```python
from build123d import *

# Parameters (mm, degrees)
BOSS_EXTRUDE1_DEPTH = 25
SKETCH2_OUTSIDE_W   = 63.85
SKETCH2_OUTSIDE_H   = 61.22
SKETCH2_OUTSIDE_R   = 8.5
CUT_EXTRUDE1_DEPTH  = 25
CUT_EXTRUDE1_DRAFT  = -35
SKETCH3_R           = 6
BOSS_EXTRUDE2_DEPTH = 110
SKETCH4_R           = 4
BOSS_EXTRUDE3_DEPTH = 6


with BuildPart() as part:
    # Sketch1 → Boss-Extrude1 (new body)
    with BuildSketch(Plane(origin=(0, 0, 0), x_dir=(1, 0, 0), z_dir=(0, 1, 0))):
        Polygon((9.814954576, 0), (4.907477288, 8.5), (-4.907477288, 8.5), (-9.814954576, 0), (-4.907477288, -8.5), (4.907477288, -8.5), align=None)
    extrude(amount=-BOSS_EXTRUDE1_DEPTH)


with BuildPart() as cut_extrude1_tool:
    # Sketch2 outside → Cut-Extrude1 (with draft: the straight prism first)
    with BuildSketch(Plane(origin=(0, 0, 0), x_dir=(1, 0, 0), z_dir=(0, 1, 0))):
        Rectangle(SKETCH2_OUTSIDE_W, SKETCH2_OUTSIDE_H)
        Circle(SKETCH2_OUTSIDE_R, mode=Mode.SUBTRACT)
    extrude(amount=-CUT_EXTRUDE1_DEPTH)
    # Cut-Extrude1: the draft: its side faces are tilted about the plane it starts from
    cut_extrude1_sides = [cut_extrude1_tool.faces().sort_by_distance(p)[0] for p in [
        (0, -12.5, 30.61),
        (31.925, -12.5, 0),
        (0, -12.5, -30.61),
        (-31.925, -12.5, 0),
        (-8.5, -12.5, 0),
    ]]
    draft(cut_extrude1_sides, Plane(origin=(0, 0, 0), x_dir=(1, 0, 0), z_dir=(0, 1, 0)), CUT_EXTRUDE1_DRAFT)


with BuildPart() as part_1:
    add(part.part)

    # Cut-Extrude1: cut by cut_extrude1_tool
    add(cut_extrude1_tool.part, mode=Mode.SUBTRACT)

    # Sketch3 → Boss-Extrude2 (add)
    with BuildSketch(Plane.XZ.offset(25)):
        with Locations(Location((0, 0, 0), (0, 0, 90))):
            Circle(SKETCH3_R)
    extrude(amount=BOSS_EXTRUDE2_DEPTH)

    # Sketch4 → Boss-Extrude3 (add)
    with BuildSketch(Plane.XZ.offset(135)):
        with Locations(Location((0, 0, 0), (0, 0, 270))):
            Circle(SKETCH4_R)
    extrude(amount=BOSS_EXTRUDE3_DEPTH)

    # Boss-Extrude4 cone 1 section (through the dimple's axis) → Boss-Extrude4 (revolve)
    with BuildSketch(Plane(origin=(0, -141, 0), x_dir=(0, 0, 1), z_dir=(1, 0, 0))):
        Polygon((0, 0), (4, 0), (0, 4), align=None)
    revolve(axis=Axis((0, -141, 0), (0, -1, 0)))


solid = part_1.part
```
Read the model definition and answer for the solid it produces. Units are mm, in the model's axes. A direction names the side the tool comes from. Give positions to 0.01 mm unless a question says otherwise; leave off trailing zeros. Write each loop counter-clockwise with the first axis right and the second up, starting at its lowest first coordinate (ties: lowest second). Pieces come first, ordered by that corner, then holes. Notation, with made-up numbers: (-20.5, -17.5) - (-10.5, -17.5) arc R22 ccw to (-10.5, 15.5) - close; hole circle Ø3 at (-35.75, -40). An arc over 180 degrees is marked (long way). Write item = value, one per line. Start each with the question number.
Item 1: Find section A-A (y = -18). Give the vertices of the cut face in (x, z), then the cut area to 3 significant figures.
Item 2: Find the intervals of material crossed by probe 1 along Y at (x, z) = (-0.5, -5.25); probe 2 along Y at (x, z) = (1.25, -7.5); probe 3 along Z at (x, y) = (-0.25, -50.5), in increasing order. Write a range as [from, to].
Item 3: Find section B-B (y = -84.5). Give the vertices of the cut face in (x, z), then the cut area to 3 significant figures.
Item 4: A tool of negligible diameter and unlimited length cuts with its end or side. For faces 1 (the conical face through (4.4, -0.4, -7.6)), 2 (the flat face through (2, -25, -6)), from which of +Z, -Z, +X, -X, +Y, -Y can it reach the whole face along a straight path? Write none if from no direction.
Item 5: Each of these flat-tipped pins is pushed along its axis until it touches: P1, Ø4, axis at x = 3, z = -2, coming from the -Y side; P2, Ø10, axis at x = -7.5, z = -1, coming from the -Y side; P3, Ø6, axis at x = 0.5, z = -2.5, coming from the -Y side; P4, Ø3, axis at x = 2, y = -36.5, coming from the +Z side. Where does it stop, or does it pass through?
Response:
q1.outline = (-9.81, 0) - (-4.91, -8.5) - (4.91, -8.5) - (9.81, 0) - (4.91, 8.5) - (-4.91, 8.5) - close
q1.area = 250 mm²
q2.probe_1 = [-135, 0]
q2.probe_2 = [-25, 0]
q2.probe_3 = [-5.99, 5.99]
q3.outline = circle Ø12 at (0, 0)
q3.area = 113 mm²
q4.face_1 = -Z, +X, +Y
q4.face_2 = -Y
q5.P1 = -143.39
q5.P2 = -142.43
q5.P3 = -145
q5.P4 = 5.98
